Source: three-view drawing plus pictorial views. Frame: mm from the lowest corner of the part. A direction names the side the tool comes from. Round coordinates to 2 decimals unless told otherwise and drop trailing zeros. Write each loop counter-clockwise with the first axis right and the second up, starting at its lowest first coordinate (ties: lowest second). Pieces come first, ordered by that corner, then holes. Notation, with made-up numbers: M 4.25,60.25 L 62.25,60.25 A16 ccw 62.25,81.25 Z; hole C -18,19 d11. An arc over 180 degrees is marked long. Answer in a Markdown table with one row per item.
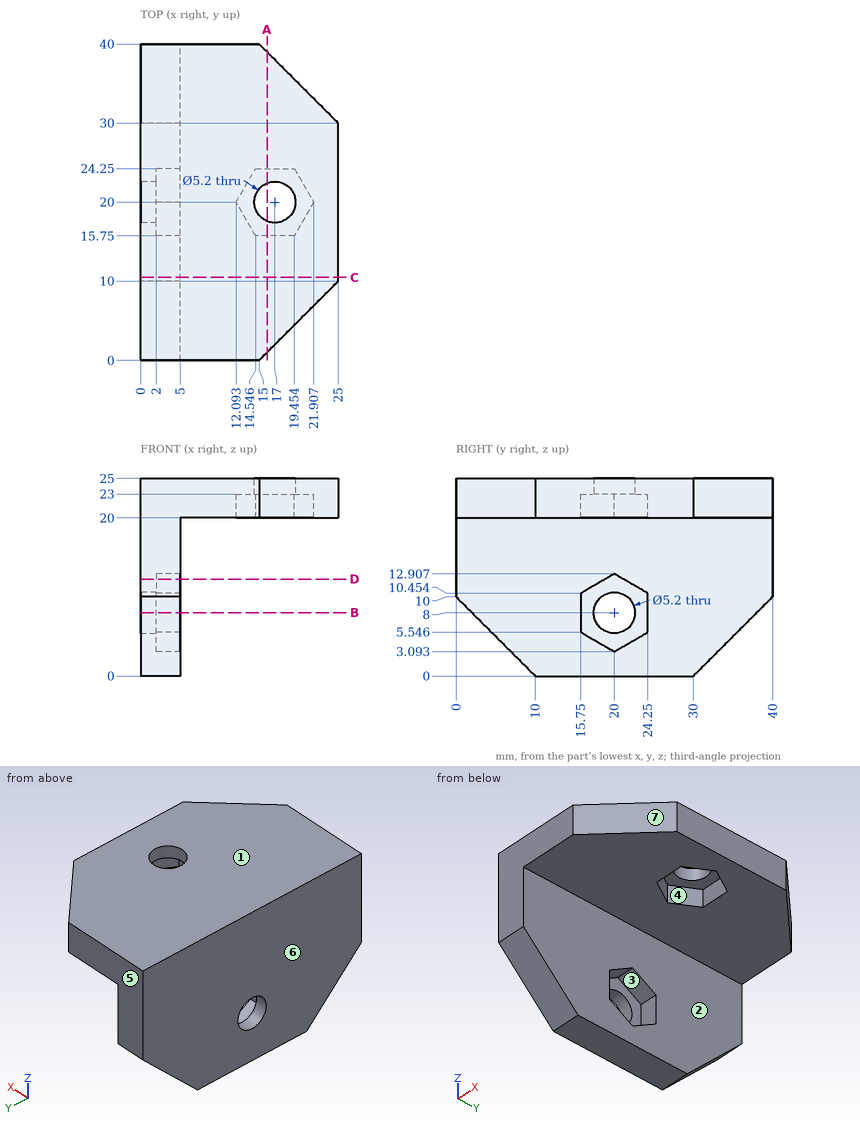
Q1. Section B-B (z = 8). Return loops of the section in (x, y).
Solutions:
| item | result |
|---|---|
| outline | M 0,2 L 5,2 L 5,15.75 L 2,15.75 L 2,17.4 L 0,17.4 Z; M 0,22.6 L 2,22.6 L 2,24.25 L 5,24.25 L 5,38 L 0,38 Z |
Q2. Contact query for flat-ended pins moving along their axis: pin 1 Ø4 at (y, z) = (20, 9) entering from +X; pin 2 Ø1.5 at (x, z) = (17.5, 21) entering from +Y; pin 3 Ø6 at (x, y) = (15, 26) entering from -Z. Output: stop coordinate, or through.
Solutions:
| item | result |
|---|---|
| pin 1 | stops at x = 2 |
| pin 2 | stops at y = 38.25 |
| pin 3 | stops at z = 20 |
Q3. Pull-direction query (X, two-part tool) for the marked faces 4, 5, 6 and 7; classes: pulls with the +X half, pulls with the -X half, needs draft (parallel to the pull), parting line crosses it, or undercut.
Solutions:
| item | result |
|---|---|
| face 4 | undercut |
| face 5 | needs draft |
| face 6 | pulls with the -X half |
| face 7 | pulls with the +X half |
Q4. Section D-D (z = 12.25). Return loops of the section in (x, y).
Solutions:
| item | result |
|---|---|
| outline | M 0,0 L 5,0 L 5,18.86 L 2,18.86 L 2,21.14 L 5,21.14 L 5,40 L 0,40 Z |
Q5. Access query for the marked faces 1, 2 and 3. Directions: +Z, -Z, +X, -X, +Y, -Y. A direction counts if a zero-diameter tool reaches every point of the face in a straight line with its end or side. Return the directions, or none.
Solutions:
| item | result |
|---|---|
| face 1 | +Z, +X, -X, +Y, -Y |
| face 2 | -Z, +X, +Y, -Y |
| face 3 | +X |
Q6. Material intervals for probe 1 along Z at (x, y) = (0.9, 20); probe 2 along Z at (x, y) = (10.75, 17); probe 3 along Y at (x, z) = (0.4, 8), sorted ascending.
Solutions:
| item | result |
|---|---|
| probe 1 | z = 0 to 5.4, 10.6 to 25 |
| probe 2 | z = 20 to 25 |
| probe 3 | y = 2 to 17.4, 22.6 to 38 |
Q7. Section C-C (y = 10.5). Return loops of the section in (x, z).
Solutions:
| item | result |
|---|---|
| outline | M 0,0 L 5,0 L 5,20 L 25,20 L 25,25 L 0,25 Z |
Q8. Section A-A (x = 16). Return loops of the section in (y, z).
Solutions:
| item | result |
|---|---|
| outline | M 1,20 L 15.75,20 L 15.75,23 L 17.6,23 L 17.6,25 L 1,25 Z; M 22.4,23 L 24.25,23 L 24.25,20 L 39,20 L 39,25 L 22.4,25 Z |
